For this review, take the finished solid that the model builds, in its own axes (mm). A direction names the side the tool comes from. Round coordinates to 2 decimals unless told otherwise and drop trailing zeros. Order: outer loops, then holes, each group sorted by start corner. A loop starts at its lowest first (then second) coordinate and runs counter-clockwise, first axis right, second up. Notation, with made-up numbers: (56.25, 29.5) - (74.25, 29.5) arc R38 ccw to (74.25, 67.5) - close; hole circle Ø4 at (81, 9.5). An arc over 180 degrees is marked (long way). Write each question's results on one line, items separated by ' | '. Start each with the question number.
(1) For L1, parallel to Y at x = 450, z = 5; L2, parallel to Z at x = 143.5, y = 671, list the stretches that pass through material, from the lowest coordinate up. Write a range as from..to.
(2) Insertion check: pin 1 Ø8 at (y, z) = (410.5, 4.5) entering from -X; pin 2 Ø3 at (x, z) = (650, 7) entering from +Y; pin 3 Ø3 at (x, z) = (450.5, 5) entering from -Y. Each pin has a flat end and moves straight along its axis. Give the tip position at first contact, or say it passes through.
(3) Draft analysis for pull direction Y (two halves, no side actions). For faces 1 (the cylindrical face through (23.846, 7.509, 798.8)), 2 (the flat face through (-6, -5, 10)), state which applies: pulls with the +Y half, pulls with the -Y half, needs draft (parallel to the pull), parting line crosses it, or undercut.
(4) Take a section at B-B, the plane y = 300. Give the boundary of the cut face in (x, z), plus the area to 3 significant figures.
(5) Take a section at A-A, the plane x = 450. Give the boundary of the cut face in (y, z), plus the area to 3 significant figures.
(6) Take a section at C-C, the plane z = 1175. Give the boundary of the cut face in (x, y), plus the area to 3 significant figures.
(7) For faces 3 (the cylindrical face through (11.5, 877.8, 798.8)), 4 (the flat face through (900, 900, 1610)), list the 3-axis set-ups (+Z, -Z, +X, -X, +Y, -Y) from which the entire face can be reached by the end or side of a thin tool; tool diameter is ignored.
```python
from build123d import *

# Parameters (mm, degrees)
F0_W     = 900
F0_H     = 900
F1_DEPTH = 10
F2_R     = 25
F3_DEPTH = 1600
F4_R     = 375
F5_DEPTH = 10.001


with BuildPart() as f1:
    # F0 (on Top) → F1 (new body)
    with BuildSketch(Plane.XY):
        with Locations((450, 450)):
            Rectangle(F0_W, F0_H)
    extrude(amount=F1_DEPTH)

    # F2 (on face) → F3 (join)
    with BuildSketch(Plane.XY.offset(10)):
        Circle(F2_R)
        with Locations((0, 900)):
            Circle(F2_R)
        with Locations((900, 900)):
            Circle(F2_R)
        with Locations((900, 0)):
            Circle(F2_R)
    extrude(amount=F3_DEPTH)

    # F4 (on face) → F5 (cut, through all)
    with BuildSketch(Plane.XY.offset(10)):
        with Locations((450, 450)):
            Circle(F4_R)
    extrude(amount=-F5_DEPTH, mode=Mode.SUBTRACT)


solid = f1.part
```
Results below:
1) L1: y = 0..75, 825..900 | L2: z = 0..10
2) pin 1: stops at x = 0 | pin 2: stops at y = 900 | pin 3: stops at y = 0
3) face 1: undercut | face 2: needs draft
4) outline: (0, 0) - (106.31, 0) - (106.31, 10) - (0, 10) - close; (793.69, 0) - (900, 0) - (900, 10) - (793.69, 10) - close | area: 2,130 mm^2
5) outline: (0, 0) - (75, 0) - (75, 10) - (0, 10) - close; (825, 0) - (900, 0) - (900, 10) - (825, 10) - close | area: 1,500 mm^2
6) outline: circle Ø50 at (0, 0); circle Ø50 at (0, 900); circle Ø50 at (900, 0); circle Ø50 at (900, 900) | area: 7,850 mm^2
7) face 3: +Z | face 4: +Z, +X, -X, +Y, -Y
